Read the model definition and answer for the solid it produces. Units are mm, in the model's axes. A direction names the side the tool comes from. Coordinates: 2 decimals unless noted, no trailing zeros. Loops run counter-clockwise (first coordinate to the right, second up) from the corner with the lowest first, then second, coordinate; pieces in that order, holes last. Notation, with made-up numbers: (43, 87.5) -> (97, 87.5) arc R26 ccw to (97, 124.5) -> close; hole circle Ø6 at (31.25, -19). An arc over 180 degrees is marked (long way). One line per question, with ' | ' between items. Start each with the question number.
```python
from build123d import *

# Parameters (mm, degrees)
F1_DEPTH = 15.494
F2_R     = 5.08
F4_DEPTH = 15.495


# Not quite as in the source:
# - a feature names something its author has since deleted; it is built from what else it names


with BuildPart() as f1:
    # F0 (on Top) → F1 (new body)
    with BuildSketch(Plane.XY):
        with BuildLine():
            ThreePointArc((-10.8447933041, 7.1841250258), (-28.0007995808, 9.0295397064), (-44.9371226132, 12.3303076252))
            Line((-44.9371226132, 12.3303076252), (-44.9371226132, -11.5082878619))
            ThreePointArc((-44.9371226132, -11.5082878619), (-28.2764136106, -8.174493828), (-11.391166434, -6.2819202055))
            ThreePointArc((-11.391166434, -6.2819202055), (-12.9978101968, 0.5273748986), (-10.8447933041, 7.1841250258))
        make_face()
        with BuildLine():
            ThreePointArc((10.9930542238, 6.9551386059), (0.1363965549, 13.007789596), (-10.8447933041, 7.1841250258))
            ThreePointArc((-10.8447933041, 7.1841250258), (0.0710380129, 6.7747130853), (10.9930542238, 6.9551386059))
        make_face()
        with BuildLine():
            ThreePointArc((10.9930542238, 6.9551386059), (0.0710380129, 6.7747130853), (-10.8447933041, 7.1841250258))
            ThreePointArc((-10.8447933041, 7.1841250258), (-12.9978101968, 0.5273748986), (-11.391166434, -6.2819202055))
            ThreePointArc((-11.391166434, -6.2819202055), (0.0626903929, -5.8267272063), (11.5236895742, -6.035376773))
            ThreePointArc((11.5236895742, -6.035376773), (12.6318479257, -3.1076698953), (13.0085046871, 0))
            ThreePointArc((13.0085046871, 0), (12.4944866159, 3.6206350823), (10.9930542238, 6.9551386059))
        make_face()
        with BuildLine():
            ThreePointArc((11.5236895742, -6.035376773), (0.0626903929, -5.8267272063), (-11.391166434, -6.2819202055))
            ThreePointArc((-11.391166434, -6.2819202055), (0.1399518192, -13.0077518305), (11.5236895742, -6.035376773))
        make_face()
        with BuildLine():
            ThreePointArc((49.3212305009, 12.3303076252), (30.2859906696, 8.7239574701), (10.9930542238, 6.9551386059))
            ThreePointArc((10.9930542238, 6.9551386059), (12.4944866159, 3.6206350823), (13.0085046871, 0))
            ThreePointArc((13.0085046871, 0), (12.6318479257, -3.1076698953), (11.5236895742, -6.035376773))
            ThreePointArc((11.5236895742, -6.035376773), (30.5547762597, -7.8580173956), (49.3212305009, -11.5082878619))
            Line((49.3212305009, -11.5082878619), (49.3212305009, 12.3303076252))
        make_face()
    extrude(amount=F1_DEPTH)

    # F2
    f2_edges = [f1.edges().sort_by_distance(p)[0] for p in [
        (-44.937123, 0.41101, 15.494),
        (49.321231, 0.41101, 15.494),
        (-44.937123, 0.41101, 0),
        (49.321231, 0.41101, 0),
        (-44.937123, 12.330308, 7.747),
        (-44.937123, -11.508288, 7.747),
        (49.321231, -11.508288, 7.747),
        (49.321231, 12.330308, 7.747),
    ]]
    fillet(f2_edges, radius=F2_R)

    # F3 (on face) → F4 (cut, through all)
    with BuildSketch(Plane.XY.offset(15.494)):
        Polygon((3.9274184965, -2.2674961262), (3.9274184965, 2.2674961262), (0, 4.5349922523), (-3.9274184965, 2.2674961262), (-3.9274184965, -2.2674961262), (0, -4.5349922523), align=None)
    extrude(amount=-F4_DEPTH, mode=Mode.SUBTRACT)


solid = f1.part
```
(1) Section A-A on y = -0.75 is taken. Write down the section's boundary in (x, z).
(2) Section D-D on x = 23.5 is taken. Write down the section's boundary in (y, z).
(3) Section B-B on z = 2.5 is taken. Write down the section's boundary in (x, y) (1 decimal), plus the area to 3 significant figures.
(4) A tool of negligible diameter and unlimited length cuts with its end or side. For faces 1 (the cylindrical face through (-42.816, 0.278, 0.951)), 2 (the cylindrical face through (27.2, -7.4, 7.6)), 3 (the flat face through (1.991, 3.385, 7.855)), 4 (the flat face through (2, -6, 15.494)), 5 (the cylindrical face through (-24.71, 8.56, 7.64)), from which of +Z, -Z, +X, -X, +Y, -Y can it reach the whole face along a straight path? Write none if from no direction.
(5) Section C-C on z = 6.5 is taken. Write down the section's boundary in (x, y) (1 decimal).
(6) Each of these flat-tipped pins is pushed along its axis until it touches: pin 1 Ø4 at (x, z) = (-13, 7.5) entering from -Y; pin 2 Ø2 at (x, z) = (12.5, 2.5) entering from +Y; pin 3 Ø1 at (x, z) = (-23, 9) entering from -Y. Where does it stop, or does it pass through?
(7) Determine the mould class of faces 6 (the flat face through (2, -6, 0)), 7 (the cylindrical face through (0.318, 13.005, 7.639)), 8 (the flat face through (3.927, 0, 8)), 9 (the cylindrical face through (-25.357, -7.742, 7.639)) for opening direction Y: +Y half, -Y half, draft (parallel to the pull), parting line (faces both ways), or undercut.
(8) Find the intervals of material crossed by probe 1 along Y at (x, z) = (0, 9.5) (1 decimal); probe 2 along X at (y, z) = (2, 14); probe 3 along X at (y, z) = (-0.5, 5), in increasing order. Write a range as from..to.
Working result:
1) outline: (-44.94, 5.08) arc R5.08 ccw to (-39.86, 0) -> (-3.93, 0) -> (-3.93, 15.49) -> (-39.86, 15.49) arc R5.08 ccw to (-44.94, 10.41) -> close; (3.93, 0) -> (44.24, 0) arc R5.08 ccw to (49.32, 5.08) -> (49.32, 10.41) arc R5.08 ccw to (44.24, 15.49) -> (3.93, 15.49) -> close
2) outline: (-6.97, 0) -> (7.89, 0) -> (7.89, 15.49) -> (-6.97, 15.49) -> close
3) outline: (-44.2, -7.7) arc R5.1 ccw to (-38.8, -10.1) arc R197.9 cw to (-11.4, -6.3) arc R13 ccw to (11.5, -6) arc R197.9 cw to (43.2, -10.1) arc R5.1 ccw to (48.6, -7.7) -> (48.6, 8.6) arc R5.1 ccw to (43.2, 11) arc R202.3 cw to (11, 7) arc R13 ccw to (-10.8, 7.2) arc R202.3 cw to (-38.8, 11) arc R5.1 ccw to (-44.2, 8.6) -> close; hole (-3.9, -2.3) -> (0, -4.5) -> (3.9, -2.3) -> (3.9, 2.3) -> (0, 4.5) -> (-3.9, 2.3) -> close | area: 1,640 mm2
4) face 1: -Z, -X, +Y, -Y | face 2: +Z, -Z, -Y | face 3: +Z, -Z | face 4: +Z, +X, -X, +Y, -Y | face 5: +Z, -Z, +Y
5) outline: (-44.9, -5.1) arc R5.1 ccw to (-38.8, -10.1) arc R197.9 cw to (-11.4, -6.3) arc R13 ccw to (11.5, -6) arc R197.9 cw to (43.2, -10.1) arc R5.1 ccw to (49.3, -5.1) -> (49.3, 6) arc R5.1 ccw to (43.2, 11) arc R202.3 cw to (11, 7) arc R13 ccw to (-10.8, 7.2) arc R202.3 cw to (-38.8, 11) arc R5.1 ccw to (-44.9, 6) -> close; hole (-3.9, -2.3) -> (0, -4.5) -> (3.9, -2.3) -> (3.9, 2.3) -> (0, 4.5) -> (-3.9, 2.3) -> close
6) pin 1: stops at y = -6.94 | pin 2: stops at y = 7.08 | pin 3: stops at y = -7.49
7) face 6: draft | face 7: +Y half | face 8: undercut | face 9: -Y half
8) probe 1: y = -13..-4.5, 4.5..13 | probe 2: x = -43.46..-3.93, 3.93..47.84 | probe 3: x = -44.94..-3.93, 3.93..49.32
